Part print with two shaded views. Sizes in mm from the minimum x, y, z corner. Give positions to 0.01 mm unless a question says otherwise; leave off trailing zeros. Write each loop counter-clockwise with the first axis right and the second up, starting at its lowest first coordinate (ties: lowest second). Pieces come first, ordered by that corner, then holes. Notation, with made-up numbers: (40.5, 85) - (83.5, 85) arc R37 cw to (83.5, 123) - close; hole circle Ø1 at (86, 14.25). An arc over 180 degrees is marked (long way). Answer as a JSON object with one key per item and string values.
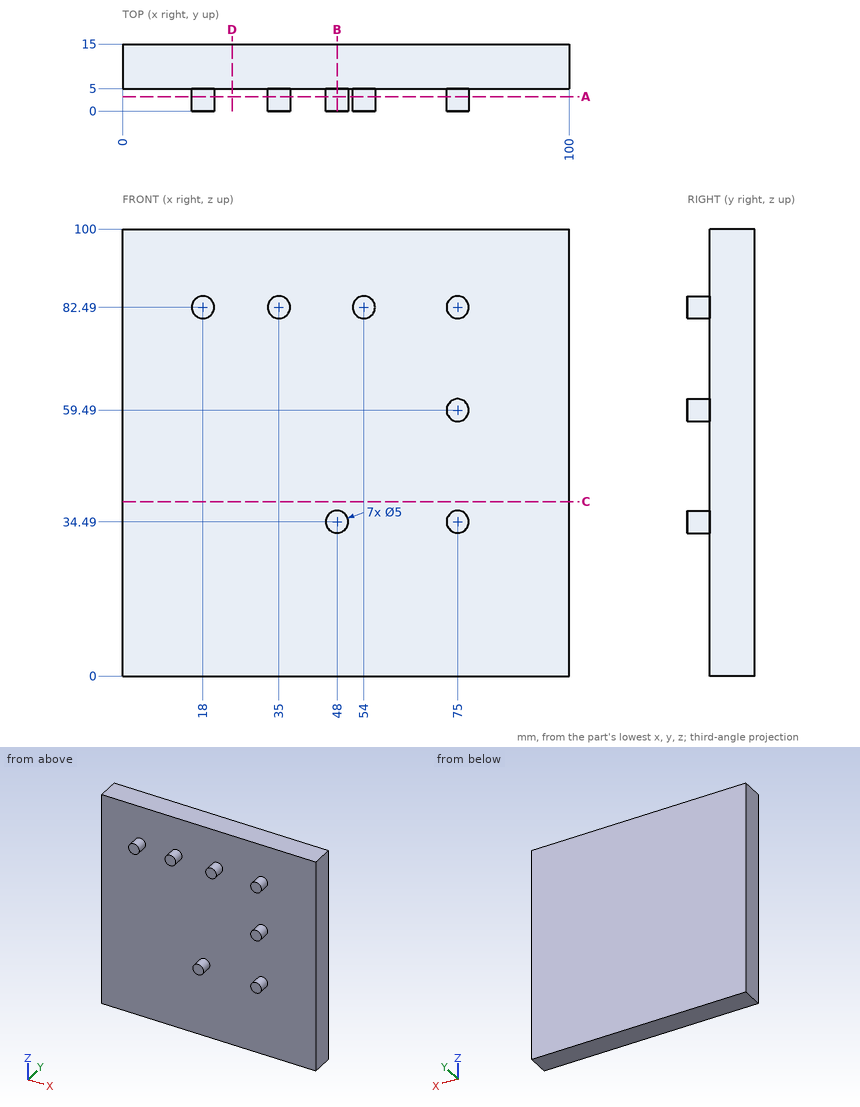
(1) Saw through at B-B, the plane x = 48. Give the cut face in (y, z), and give its area (4 significant figures).
Answer key:
{"outline": "(0, 31.99) - (5, 31.99) - (5, 0) - (15, 0) - (15, 100) - (5, 100) - (5, 36.99) - (0, 36.99) - close", "area": "1,025 mm²"}
(2) Saw through at A-A, the plane y = 3.25. Give the cut face in (x, z).
Answer key:
{"outline": "circle Ø5 at (18, 82.49); circle Ø5 at (35, 82.49); circle Ø5 at (48, 34.49); circle Ø5 at (54, 82.49); circle Ø5 at (75, 34.49); circle Ø5 at (75, 59.49); circle Ø5 at (75, 82.49)"}
(3) Flat gauge pin, fed straight in: P1, Ø5, axis at y = 5.5, z = 41.5, coming from the -X side. Where does the tip first touch, or does it go through?
Answer key:
{"P1": "stops at x = 0"}
(4) Saw through at C-C, the plane z = 39. Give the cut face in (x, y), and give its area (3 significant figures).
Answer key:
{"outline": "(0, 5) - (100, 5) - (100, 15) - (0, 15) - close", "area": "1,000 mm²"}
(5) Probe L1, parallel to X at y = 3.75, z = 81; L2, parallel to Y at x = 32, z = 60; L3, parallel to Z at x = 35.5, y = 3. List the from-to ranges inside material, lowest first. Write a range as [from, to].
Answer key:
{"L1": "x = [15.99, 20.01], [32.99, 37.01], [51.99, 56.01], [72.99, 77.01]", "L2": "y = [5, 15]", "L3": "z = [80.04, 84.94]"}
(6) Saw through at D-D, the plane x = 24.5. Give the cut face in (y, z).
Answer key:
{"outline": "(5, 0) - (15, 0) - (15, 100) - (5, 100) - close"}
